Geometry check sheet. Reference: drawing and pictorial views, mm from the part's lowest x, y, z. A direction names the side the tool comes from. Give positions to 0.01 mm unless a question says otherwise; leave off trailing zeros. Order: outer loops, then holes, each group sorted by start corner. A loop starts at its lowest first (then second) coordinate and runs counter-clockwise, first axis right, second up. Notation, with made-up numbers: (50, -18.5) - (90, -18.5) arc R6 cw to (90, -8.5) - close; hole circle Ø2 at (86.5, -9.75). An arc over 180 degrees is marked (long way). Answer as a JSON object with one key per item and string values.
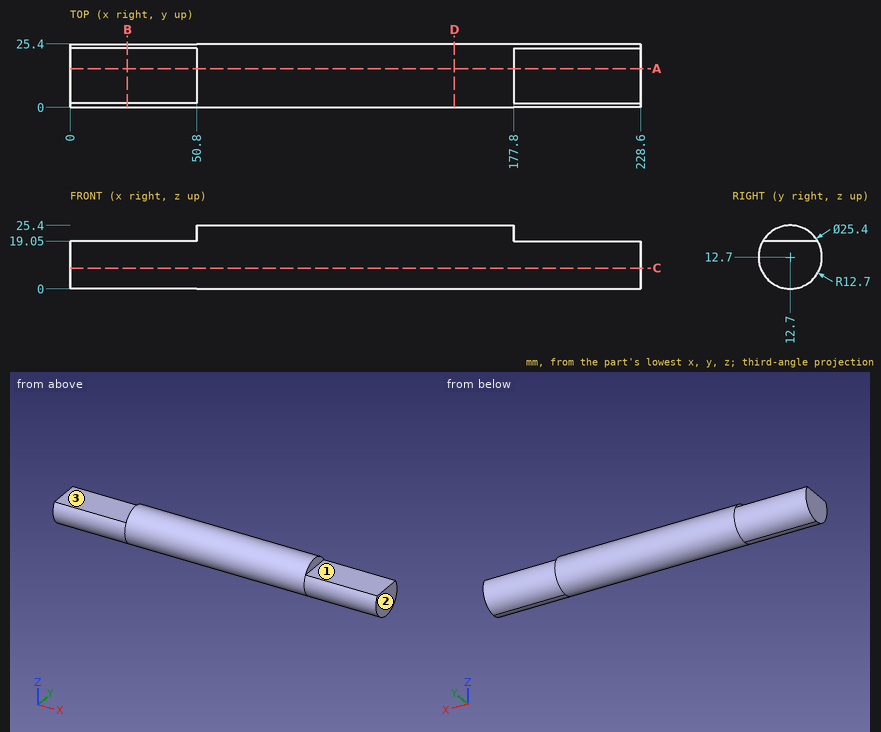
(1) Material ranges on line 1 along X through (y, z) = (12.5, 20); line 2 along Z through (x, y) = (99, 4.75); line 3 along Y through (x, z) = (16, 9.25), recorded low to high. Write a range as [from, to].
Computed values:
{"line 1": "x = [50.8, 177.8]", "line 2": "z = [2.8, 22.6]", "line 3": "y = [0.48, 24.92]"}
(2) Section check B-B (x = 23). Record the cut outline in (y, z).
Computed values:
{"outline": "(1.7, 19.05) arc R12.7 ccw (long way) to (23.7, 19.05) - close"}
(3) Section check C-C (z = 8.25). Record the cut outline in (x, y), then the cut area to 3 significant figures.
Computed values:
{"outline": "(0, 0.81) - (228.6, 0.81) - (228.6, 24.59) - (0, 24.59) - close", "area": "5,440 mm²"}
(4) Section check D-D (x = 154). Record the cut outline in (y, z), then the cut area to 3 significant figures.
Computed values:
{"outline": "circle Ø25.4 at (12.7, 12.7)", "area": "507 mm²"}
(5) Section check A-A (y = 15.5). Record the cut outline in (x, z).
Computed values:
{"outline": "(0, 0.31) - (228.6, 0.31) - (228.6, 19.05) - (177.8, 19.05) - (177.8, 25.09) - (50.8, 25.09) - (50.8, 19.05) - (0, 19.05) - close"}
(6) Access from +Z, -Z, +X, -X, +Y, -Y to the whole of each face (thin tool, end or side, straight path). Record for the marked faces 1, 2 and 3.
Computed values:
{"face 1": "+Z, +X, +Y, -Y", "face 2": "+Z, -Z, +X, +Y, -Y", "face 3": "+Z, -X, +Y, -Y"}
(7) Gauge pin test, flat ends, axial feed: pin 1 Ø6.5 at (x, y) = (214, 15.5) entering from +Z; pin 2 Ø6 at (x, z) = (58.5, 21.5) entering from -Y; pin 3 Ø5 at (x, y) = (85.5, 10) entering from +Z. Record the tip position at first contact, or that the pin passes through.
Computed values:
{"pin 1": "stops at z = 19.05", "pin 2": "stops at y = 1.4", "pin 3": "stops at z = 25.4"}
